from build123d import *

# Parameters (mm, degrees)
F0_R     = 2
F1_DEPTH = 5
F2_R     = 1
F3_R     = 1
F4_DEPTH = 10


with BuildPart() as f1:
    # F0 (on Top) → F1 (new body)
    with BuildSketch(Plane.XY):
        Polygon((0, 22.7317288518), (0, 0), (10, 0), (10, 22.7317288518), (7.5, 22.7317288518), (5, 22.7317288518), (2.5, 22.7317288518), align=None)
        with Locations((4.8133912496, 4.4267121702)):
            Circle(F0_R, mode=Mode.SUBTRACT)
        with Locations((4.8133912496, 17.8769808263)):
            Circle(F0_R, mode=Mode.SUBTRACT)
        with BuildLine():
            Line((2.5, 52.7317288518), (2.5, 22.7317288518))
            Line((2.5, 22.7317288518), (5, 22.7317288518))
            Line((5, 22.7317288518), (5, 51.2317288518))
            ThreePointArc((5, 51.2317288518), (3.9393398282, 51.67106868), (3.5, 52.7317288518))
            ThreePointArc((3.5, 52.7317288518), (3.4744103207, 53.6926062484), (3.3977138284, 54.6507596031))
            ThreePointArc((3.3977138284, 54.6507596031), (2.7355226399, 53.7910410275), (2.5, 52.7317288518))
        make_face()
        with BuildLine():
            Line((5, 22.7317288518), (7.5, 22.7317288518))
            Line((7.5, 22.7317288518), (7.5, 52.7317288518))
            ThreePointArc((7.5, 52.7317288518), (7.2072929768, 53.9055506928), (6.3977138284, 54.8045038164))
            ThreePointArc((6.3977138284, 54.8045038164), (6.4744129083, 53.7693774574), (6.5, 52.7317288518))
            ThreePointArc((6.5, 52.7317288518), (6.0606601718, 51.67106868), (5, 51.2317288518))
            Line((5, 51.2317288518), (5, 22.7317288518))
        make_face()
        with BuildLine():
            ThreePointArc((3.5, 52.7317288518), (3.9393398282, 51.67106868), (5, 51.2317288518))
            Line((5, 51.2317288518), (5, 52.7317288518))
            ThreePointArc((5, 52.7317288518), (4.960003557, 53.9817288518), (4.8401778569, 55.226614998))
            ThreePointArc((4.8401778569, 55.226614998), (4.073091813, 55.053547366), (3.3977138284, 54.6507596031))
            ThreePointArc((3.3977138284, 54.6507596031), (3.4744103207, 53.6926062484), (3.5, 52.7317288518))
        make_face()
        with BuildLine():
            Line((5, 52.7317288518), (5, 51.2317288518))
            ThreePointArc((5, 51.2317288518), (6.0606601718, 51.67106868), (6.5, 52.7317288518))
            ThreePointArc((6.5, 52.7317288518), (6.4744129083, 53.7693774574), (6.3977138284, 54.8045038164))
            ThreePointArc((6.3977138284, 54.8045038164), (5.6539406843, 55.144685872), (4.8401778569, 55.226614998))
            ThreePointArc((4.8401778569, 55.226614998), (4.960003557, 53.9817288518), (5, 52.7317288518))
        make_face()
        with BuildLine():
            ThreePointArc((-28.0449956093, 40.7368995467), (-21.8583839955, 69.2405574995), (3.3977138284, 54.6507596031))
            ThreePointArc((3.3977138284, 54.6507596031), (4.073091813, 55.053547366), (4.8401778569, 55.226614998))
            ThreePointArc((4.8401778569, 55.226614998), (-21.968116408, 70.8241322208), (-30.1189319968, 40.8987017286))
            ThreePointArc((-30.1189319968, 40.8987017286), (-29.0493590182, 41.2357199074), (-28.0449956093, 40.7368995467))
        make_face()
        with BuildLine():
            ThreePointArc((4.8401778569, 55.226614998), (5.6539406843, 55.144685872), (6.3977138284, 54.8045038164))
            ThreePointArc((6.3977138284, 54.8045038164), (-22.9963973106, 72.0173965367), (-30.2870642065, 38.7436287659))
            ThreePointArc((-30.2870642065, 38.7436287659), (-30.661485659, 39.856935046), (-30.1189319968, 40.8987017286))
            ThreePointArc((-30.1189319968, 40.8987017286), (-21.968116408, 70.8241322208), (4.8401778569, 55.226614998))
        make_face()
        with BuildLine():
            Line((-9.0393445759, 19.3589845332), (-28.0449956093, 40.7368995467))
            ThreePointArc((-28.0449956093, 40.7368995467), (-27.6686113105, 39.6523008448), (-28.1693945175, 38.6192298577))
            Line((-28.1693945175, 38.6192298577), (-11.1570142649, 19.4833834414))
            ThreePointArc((-11.1570142649, 19.4833834414), (-10.0724155629, 19.8597677402), (-9.0393445759, 19.3589845332))
        make_face()
        with BuildLine():
            ThreePointArc((-28.1693945175, 38.6192298577), (-27.6686113105, 39.6523008448), (-28.0449956093, 40.7368995467))
            ThreePointArc((-28.0449956093, 40.7368995467), (-29.0493590182, 41.2357199074), (-30.1189319968, 40.8987017286))
            ThreePointArc((-30.1189319968, 40.8987017286), (-29.6535936799, 40.3103418877), (-29.1660299079, 39.7402641563))
            Line((-29.1660299079, 39.7402641563), (-28.1693945175, 38.6192298577))
        make_face()
        with BuildLine():
            ThreePointArc((-30.1189319968, 40.8987017286), (-30.661485659, 39.856935046), (-30.2870642065, 38.7436287659))
            ThreePointArc((-30.2870642065, 38.7436287659), (-29.2539932195, 38.2428455589), (-28.1693945175, 38.6192298577))
            Line((-28.1693945175, 38.6192298577), (-29.1660299079, 39.7402641563))
            ThreePointArc((-29.1660299079, 39.7402641563), (-29.6535936799, 40.3103418877), (-30.1189319968, 40.8987017286))
        make_face()
        with BuildLine():
            ThreePointArc((-28.1693945175, 38.6192298577), (-29.2539932195, 38.2428455589), (-30.2870642065, 38.7436287659))
            Line((-30.2870642065, 38.7436287659), (-11.2814131731, 17.3657137524))
            ThreePointArc((-11.2814131731, 17.3657137524), (-11.6577974719, 18.4503124544), (-11.1570142649, 19.4833834414))
            Line((-11.1570142649, 19.4833834414), (-28.1693945175, 38.6192298577))
        make_face()
        with BuildLine():
            ThreePointArc((-11.4373132839, 1.3031069234), (-6.1047109197, 9.7820673373), (-9.0393445759, 19.3589845332))
            ThreePointArc((-9.0393445759, 19.3589845332), (-8.6670458513, 18.2210817301), (-9.2461191516, 17.1731775156))
            ThreePointArc((-9.2461191516, 17.1731775156), (-10.3016462873, 16.8690161197), (-11.2814131731, 17.3657137524))
            ThreePointArc((-11.2814131731, 17.3657137524), (-9.0785988115, 10.1770240522), (-13.0813924983, 3.8124900222))
            ThreePointArc((-13.0813924983, 3.8124900222), (-13.5140444405, 1.7357588655), (-11.4373132839, 1.3031069234))
        make_face()
        with BuildLine():
            ThreePointArc((-9.2461191516, 17.1731775156), (-8.6670458513, 18.2210817301), (-9.0393445759, 19.3589845332))
            ThreePointArc((-9.0393445759, 19.3589845332), (-10.0724155629, 19.8597677402), (-11.1570142649, 19.4833834414))
            Line((-11.1570142649, 19.4833834414), (-10.1603788745, 18.3623491428))
            ThreePointArc((-10.1603788745, 18.3623491428), (-9.6820476982, 17.7840633382), (-9.2461191516, 17.1731775156))
        make_face()
        with BuildLine():
            ThreePointArc((-11.1570142649, 19.4833834414), (-11.6577974719, 18.4503124544), (-11.2814131731, 17.3657137524))
            ThreePointArc((-11.2814131731, 17.3657137524), (-10.3016462873, 16.8690161197), (-9.2461191516, 17.1731775156))
            ThreePointArc((-9.2461191516, 17.1731775156), (-9.6820476982, 17.7840633382), (-10.1603788745, 18.3623491428))
            Line((-10.1603788745, 18.3623491428), (-11.1570142649, 19.4833834414))
        make_face()
    extrude(amount=F1_DEPTH)

    # F2
    f2_edges = [f1.edges().sort_by_distance(p)[0] for p in [
        (0, 22.731729, 2.5),
        (2.5, 22.731729, 2.5),
        (10, 22.731729, 2.5),
        (7.5, 22.731729, 2.5),
        (10, 0, 2.5),
        (0, 0, 2.5),
    ]]
    fillet(f2_edges, radius=F2_R)

    # F3 (on face) → F4 (cut, through all)
    with BuildSketch(Plane.YZ.offset(10)):
        with Locations((11.3658644259, 2.5)):
            Circle(F3_R)
    extrude(amount=-F4_DEPTH, mode=Mode.SUBTRACT)


solid = f1.part
Geometry: final body of the model. Coordinates: model frame, mm. A direction names the side the tool comes from. Round coordinates to 2 decimals unless told otherwise and drop trailing zeros. Loops run counter-clockwise (first coordinate to the right, second up) from the corner with the lowest first, then second, coordinate; pieces in that order, holes last. Notation, with made-up numbers: (-2, 75) -> (18, 75) arc R13 cw to (18, 88) -> close; hole circle Ø2 at (73, 1). An arc over 180 degrees is marked (long way). One line per question, with ' | ' between items. Start each with the question number.
1. Mould query, pull axis Z, two halves, no side actions, for faces 6 (the face through (5.07, 10.367, 2.544)), 7 (the face through (-9.065, 10.285, 2.465)), 8 (the face through (4, 34, 0)). Classes: pulls with the +Z half, pulls with the -Z half, needs draft (parallel to the pull), parting line crosses it, or undercut.
2. Section B-B on z = 2.5. Output: boundary loops of the cut face in (x, y) (1 decimal).
3. Section A-A on x = 5. Output: boundary loops of the cut face in (y, z).
4. Line query: line 1 along Y through (x, z) = (-12, 4); line 2 along Y through (x, z) = (-12.5, 3.95); line 3 along X through (y, z) = (4.5, 2.8). Output: solid intervals per line, ascending. Write a range as [from, to].
5. Contact query for flat-ended pins moving along their axis: pin 1 (1.5 mm diameter, centred on y = 49, z = 1, fed in from +X); pin 2 (1.5 mm diameter, centred on y = 32, z = 3, fed in from -X); pin 3 (0.6 mm diameter, centred on x = 8.5, z = 3, fed in from +Y). Output: stop coordinate, or through.
6. Section C-C on x = -7.5. Output: boundary loops of the cut face in (y, z), and give its area (3 significant figures).
7. Set-up query: faces 1 (the face through (4, 34, 5)), 2 (the face through (7.5, 38, 2)), 3 (the face through (0, 12, 1)), 4 (the face through (10, 11, 1)), 5 (the face through (-18.41, 29.9, 2.46)). Return all of +Z, -Z, +X, -X, +Y, -Y with unobstructed straight access to the full face (end or side cutting, diameter ignored); none if empty.
8. Section D-D on x = -21. Output: boundary loops of the cut face in (y, z), and give its area (3 significant figures).
Returned:
1) face 6: undercut | face 7: needs draft | face 8: pulls with the -Z half
2) outline: (-30.3, 38.7) -> (-11.3, 17.4) arc R9 cw to (-13.1, 3.8) arc R1.5 ccw to (-11.4, 1.3) arc R12 ccw to (-9, 19.4) -> (-28, 40.7) arc R18.1 cw (long way) to (3.4, 54.7) arc R2.5 ccw to (2.5, 52.7) -> (2.5, 23.7) arc R1 cw to (1.5, 22.7) -> (1, 22.7) arc R1 ccw to (0, 21.7) -> (0, 12.4) -> (10, 12.4) -> (10, 21.7) arc R1 ccw to (9, 22.7) -> (8.5, 22.7) arc R1 cw to (7.5, 23.7) -> (7.5, 52.7) arc R2.5 ccw to (6.4, 54.8) arc R21.1 ccw (long way) to start; (0, 1) arc R1 ccw to (1, 0) -> (9, 0) arc R1 ccw to (10, 1) -> (10, 10.4) -> (0, 10.4) -> close; hole circle Ø4 at (4.8, 4.4); hole circle Ø4 at (4.8, 17.9)
3) outline: (0, 0) -> (2.44, 0) -> (2.44, 5) -> (0, 5) -> close; (6.42, 0) -> (15.89, 0) -> (15.89, 5) -> (6.42, 5) -> close; (19.87, 0) -> (60.54, 0) -> (60.54, 5) -> (19.87, 5) -> close; hole circle Ø2 at (11.37, 2.5)
4) line 1: y = [1.08, 4.64], [18.17, 22.69], [70.6, 73.63] | line 2: y = [1.08, 4.23], [18.74, 23.25], [70.67, 73.68] | line 3: x = [-12.16, -8.15], [0, 2.81], [6.81, 10]
5) pin 1: stops at x = 7.5 | pin 2: stops at x = -24.96 | pin 3: stops at y = 22.78
6) outline: (5.55, 0) -> (17.18, 0) -> (17.18, 5) -> (5.55, 5) -> close; (69.35, 0) -> (72.57, 0) -> (72.57, 5) -> (69.35, 5) -> close | area: 74.3 mm2
7) face 1: +Z, +X, -X, +Y, -Y | face 2: +Z, -Z, +X, +Y | face 3: +Z, -Z, -Y | face 4: +Z, -Z, +X, +Y, -Y | face 5: +Z, -Z
8) outline: (28.3, 0) -> (32.81, 0) -> (32.81, 5) -> (28.3, 5) -> close; (69.59, 0) -> (72.77, 0) -> (72.77, 5) -> (69.59, 5) -> close | area: 38.5 mm2
